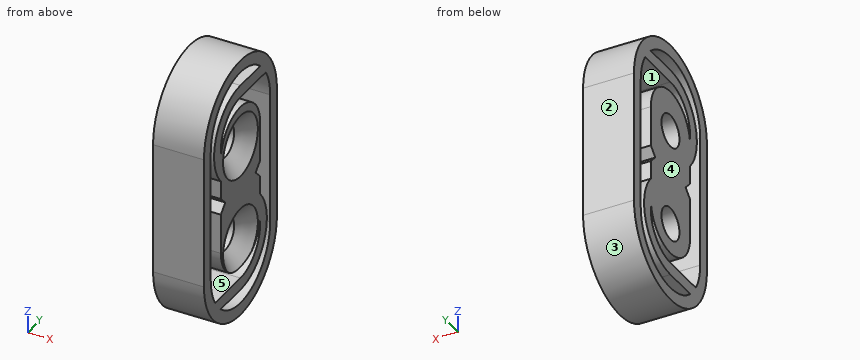
from build123d import *

# Parameters (mm, degrees)
BOSS_EXTRUDE2_DEPTH = 5
SKETCH4_R           = 1.6
CUT_EXTRUDE1_DEPTH  = 10
CHAMFER1_SIZE       = 1.5


with BuildPart() as part:
    # Sketch2 → Boss-Extrude2 (new body)
    with BuildSketch(Plane.YZ):
        with BuildLine():
            Line((-6.472145094, 6.496243265), (-6.472145094, -6.503756735))
            ThreePointArc((-6.472145094, -6.503756735), (0.027854906, -13.003756735), (6.527854906, -6.503756735))
            Line((6.527854906, -6.503756735), (6.527854906, 6.496243265))
            ThreePointArc((6.527854906, 6.496243265), (0.027854906, 12.996243265), (-6.472145094, 6.496243265))
        make_face()
        with BuildLine():
            Line((-5.272145094, 6.496243265), (-5.272145094, -6.503756735))
            ThreePointArc((-5.272145094, -6.503756735), (-5.076205272, -7.931541625), (-4.502873512, -9.253756735))
            Line((-4.502873512, -9.253756735), (0.027854906, -9.253756735))
            ThreePointArc((0.027854906, -9.253756735), (2.673606218, -8.045044583), (3.491956522, -5.253756735))
            ThreePointArc((3.491956522, -5.253756735), (-0.222788612, -8.244770603), (-3.472145094, -4.753756735))
            Line((-3.472145094, -4.753756735), (-3.472145094, -0.803756735))
            Line((-3.472145094, -0.803756735), (-2.672145094, -0.003756735))
            Line((-2.672145094, -0.003756735), (-3.472145094, 0.796243265))
            Line((-3.472145094, 0.796243265), (-3.472145094, 2.609365837))
            ThreePointArc((-3.472145094, 2.609365837), (-4.263608941, 7.662838695), (0.027854906, 10.446243265))
            Line((0.027854906, 10.446243265), (3.561620603, 10.446243265))
            ThreePointArc((3.561620603, 10.446243265), (-2.135596249, 11.334577596), (-5.272145094, 6.496243265))
        make_face(mode=Mode.SUBTRACT)
        with BuildLine():
            Line((4.558583325, 9.246243265), (0.027854906, 9.246243265))
            ThreePointArc((0.027854906, 9.246243265), (-2.617896405, 8.037531112), (-3.436246709, 5.246243265))
            ThreePointArc((-3.436246709, 5.246243265), (0.278498425, 8.237257133), (3.527854906, 4.746243265))
            Line((3.527854906, 4.746243265), (3.527854906, 0.796243265))
            Line((3.527854906, 0.796243265), (2.727854906, -0.003756735))
            Line((2.727854906, -0.003756735), (3.527854906, -0.803756735))
            Line((3.527854906, -0.803756735), (3.527854906, -2.616879307))
            ThreePointArc((3.527854906, -2.616879307), (4.319318754, -7.670352166), (0.027854906, -10.453756735))
            Line((0.027854906, -10.453756735), (-3.50591079, -10.453756735))
            ThreePointArc((-3.50591079, -10.453756735), (2.191306062, -11.342091066), (5.327854906, -6.503756735))
            Line((5.327854906, -6.503756735), (5.327854906, 6.496243265))
            ThreePointArc((5.327854906, 6.496243265), (5.131915085, 7.924028155), (4.558583325, 9.246243265))
        make_face(mode=Mode.SUBTRACT)
    extrude(amount=BOSS_EXTRUDE2_DEPTH)

    # Sketch4 → Cut-Extrude1 (cut)
    with BuildSketch(Plane.YZ.offset(5)):
        with Locations(Location((0.027854906, 4.246243265, 0), (0, 0, 270))):
            Circle(SKETCH4_R)
        with Locations(Location((0.027854906, -5.253756735, 0), (0, 0, 270))):
            Circle(SKETCH4_R)
    extrude(amount=-CUT_EXTRUDE1_DEPTH, mode=Mode.SUBTRACT)

    # Chamfer1
    # the kernel refuses this chamfer: 1.5 mm, written as the material it takes off along each edge
    with BuildSketch(Plane(origin=(5, 0.027854906, 4.246243265), x_dir=(0, 0, -1), z_dir=(0, -1, 0))) as chamfer1_piece_1:
        Polygon((1.6 + CHAMFER1_SIZE, 0), (1.6, -CHAMFER1_SIZE), (1.6, 0), align=None)
    revolve(axis=Axis((5, 0.027854906, 4.246243265), (1, 0, 0)), mode=Mode.SUBTRACT)
    with BuildSketch(Plane(origin=(5, 0.027854906, -5.253756735), x_dir=(0, 0, -1), z_dir=(0, -1, 0))) as chamfer1_piece_2:
        Polygon((1.6 + CHAMFER1_SIZE, 0), (1.6, -CHAMFER1_SIZE), (1.6, 0), align=None)
    revolve(axis=Axis((5, 0.027854906, -5.253756735), (1, 0, 0)), mode=Mode.SUBTRACT)


solid = part.part
Build history of the part. All positions in model axes, mm. Face numbers are marked on the shaded views. A direction names the side the tool comes from. Round coordinates to 2 decimals unless told otherwise and drop trailing zeros. Write each loop counter-clockwise with the first axis right and the second up, starting at its lowest first coordinate (ties: lowest second). Pieces come first, ordered by that corner, then holes. Notation, with made-up numbers: (71.5, -28) -> (91.5, -28) arc R28 ccw to (91.5, 0) -> close; hole circle Ø2 at (79.25, 8.25). An arc over 180 degrees is marked (long way). Use one line per item in the form item = value.
Q1. Band-saw the part on C-C, the plane z = -0.25. Write the cut outline in (x, y), then the cut area to 3 significant figures.
Conclusion:
outline = (0, -6.47) -> (5, -6.47) -> (5, -5.27) -> (0, -5.27) -> close; (0, -2.92) -> (5, -2.92) -> (5, 2.97) -> (0, 2.97) -> close; (0, 5.33) -> (5, 5.33) -> (5, 6.53) -> (0, 6.53) -> close
area = 41.5 mm²
Q2. Drill centre lines: L1, parallel to Y at x = 3.2, z = -2.25; L2, parallel to Y at x = 1.4, z = 4.5; L3, parallel to Y at x = 4.1, z = -7.75. Where is each one in solid material? Low to high.
Conclusion:
L1 = -6.47 to -5.27, -3.47 to 3.53, 5.33 to 6.53
L2 = -6.47 to -5.27, -4.5 to -1.55, 1.61 to 3.53, 5.33 to 6.53
L3 = -6.35 to -5.12, -1.78 to 1.84, 2.9 to 4.28, 5.18 to 6.41
Q3. Drop flat-ended pins along their axis: P1, Ø1.1, axis at x = 3, y = -2.5, coming from the -Z side; P2, Ø1.5, axis at x = 2, y = -1.5, coming from the -Z side; P3, Ø3, axis at y = -4.5, z = -2, coming from the +X side; P4, Ø2.5, axis at y = 0.03, z = -5.25, coming from the -X side. Give the stop position or say it passes through.
Conclusion:
P1 = -12.7
P2 = -12.96
P3 = 5
P4 = through
Q4. Band-saw the part on A-A, the plane z = -11. Write the cut outline in (x, y), then the cut area to 3 significant figures.
Conclusion:
outline = (0, -4.67) -> (5, -4.67) -> (5, -2.78) -> (0, -2.78) -> close; (0, 2.83) -> (5, 2.83) -> (5, 4.72) -> (0, 4.72) -> close
area = 18.9 mm²
Q5. Band-saw the part on D-D, the plane z = 10.75. Write the cut outline in (x, y), then the cut area to 3 significant figures.
Conclusion:
outline = (0, -4.89) -> (5, -4.89) -> (5, -3.13) -> (0, -3.13) -> close; (0, 3.19) -> (5, 3.19) -> (5, 4.94) -> (0, 4.94) -> close
area = 17.5 mm²
Q6. Two-plate mould, pull along Z, no slides. Class the marked faces 1, 2 and 3: released by +Z, released by -Z, zero draft, split by the parting line, or undercut.
Conclusion:
face_1 = undercut
face_2 = zero draft
face_3 = released by -Z
Q7. Band-saw the part on B-B, the plane x = 1.95. State how many separate pieces and enclosed holes the cut face has, then the cut area to 3 significant figures.
Conclusion:
separate_pieces = 1
enclosed_holes = 4
area = 194 mm²
Q8. Tool access for the marked faces 4 and 5: list every direction of +Z, -Z, +X, -X, +Y, -Y with a clear straight run to the whole face (end or side of a thin tool).
Conclusion:
face_4 = +Z, -Z, -X, +Y, -Y
face_5 = +X, -X
